Input: part model. Units: mm. Frame: model coordinates. Coordinates: 2 decimals unless noted, no trailing zeros. Order: outer loops, then holes, each group sorted by start corner. A loop starts at its lowest first (then second) coordinate and runs counter-clockwise, first axis right, second up. Notation, with made-up numbers: (-5.5, 21) -> (43.5, 21) arc R27 cw to (43.5, 42) -> close; hole circle Ø5 at (14, 78). An arc over 180 degrees is marked (long way). Answer as CSV lines item,"result".
from build123d import *

# Parameters (mm, degrees)
F1_DEPTH = 5
F3_DEPTH = 80
F5_DEPTH = 20
F6_SIZE2 = 2.3835071852
F6_SIZE  = 2


with BuildPart() as f1:
    # F0 (on Top) → F1 (new body)
    with BuildSketch(Plane.XY):
        Polygon((0, 0), (0, 50), (-15, 50), (-15, -25), (40, -25), (40, 0), align=None)
    extrude(amount=F1_DEPTH)

    # F2 (on face) → F3 (cut)
    with BuildSketch(Plane.XZ.offset(25)):
        with BuildLine():
            ThreePointArc((-15, 1), (12.4054654459, 4.3708490427), (40, 3.3891045123))
            Line((40, 3.3891045123), (40, 5))
            Line((40, 5), (-15, 5))
            Line((-15, 5), (-15, 1))
        make_face()
    extrude(amount=-F3_DEPTH, mode=Mode.SUBTRACT)

    # F4 (on face) → F5 (join)
    with BuildSketch(Plane(origin=(0, 0, 0), x_dir=(1, 0, 0), z_dir=(0, 0, -1))):
        Polygon((-17, -50), (-15, -50), (-15, 25), (40, 25), (40, 27), (-17, 27), align=None)
    extrude(amount=-F5_DEPTH)

    # F6
    f6_edges = [f1.edges().sort_by_distance(p)[0] for p in [
        (20, 0, 0),
        (0, 25, 0),
    ]]
    f6_side = f1.faces().sort_by_distance((-0.958019, 25, 0))[0]
    chamfer(f6_edges, length=F6_SIZE, length2=F6_SIZE2, reference=f6_side)


solid = f1.part
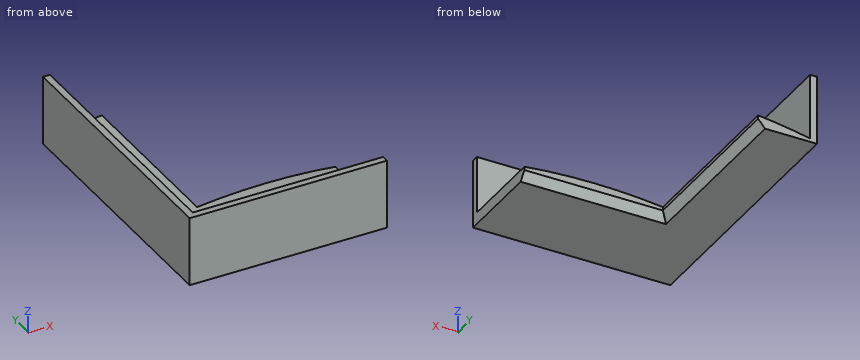
1. Cut plane A-A (y = 41). Return the cut outline in (x, z).
Findings:
outline,"(-17, 0) -> (-2, 0) -> (0, 2.38) -> (0, 3.39) arc R175 ccw to (-15, 1) -> (-15, 20) -> (-17, 20) -> close"
2. Cut plane B-B (x = 23). Return the cut outline in (y, z), plus the area to 3 significant figures.
Findings:
outline,"(-27, 0) -> (-2, 0) -> (0, 2.38) -> (0, 4.51) -> (-25, 4.51) -> (-25, 20) -> (-27, 20) -> close"
area,"150 mm2"
3. Cut plane C-C (z = 12). Return the cut outline in (x, y).
Findings:
outline,"(-17, -27) -> (40, -27) -> (40, -25) -> (-15, -25) -> (-15, 50) -> (-17, 50) -> close"
4. Contact query for flat-ended pins moving along their axis: pin 1 (2 mm diameter, centred on y = 0.5, z = 18, fed in from +X); pin 2 (0.8 mm diameter, centred on y = 36.5, z = 3, fed in from +X); pin 3 (0.6 mm diameter, centred on x = 13.5, z = 3, fed in from +Y). Output: stop coordinate, or through.
Findings:
pin 1,"stops at x = -15"
pin 2,"stops at x = 0"
pin 3,"stops at y = 0"
5. Cut plane D-D (y = -9). Return the cut outline in (x, z).
Findings:
outline,"(-17, 0) -> (40, 0) -> (40, 3.39) arc R175 ccw to (-15, 1) -> (-15, 20) -> (-17, 20) -> close"
6. Ray query, line 1 along X through (y, z) = (19.5, 8.75); line 2 along Y through (x, z) = (9.5, 10.25); line 3 along Y through (x, z) = (32.5, 3.5). Return the intervals inside material, ascending.
Findings:
line 1,"x = -17 to -15"
line 2,"y = -27 to -25"
line 3,"y = -27 to 0"
